Input: part model. Units: mm. Frame: model coordinates. A direction names the side the tool comes from. Round coordinates to 2 decimals unless told otherwise and drop trailing zeros. Write each loop counter-clockwise with the first axis right and the second up, starting at its lowest first coordinate (ties: lowest second). Pieces come first, ordered by that corner, then holes. Notation, with made-up numbers: M 30,71.25 L 89,71.25 A37 cw 89,110.25 Z; hole C 63.25,23.25 d9. An arc over 180 degrees is marked long. Answer as CSV lines item,"result". Start each with the question number.
```python
from build123d import *

# Parameters (mm, degrees)
F1_DEPTH      = 2
F2_R          = 1.663036
F3_DEPTH      = 1
F3_DEPTH_BACK = 2


with BuildPart() as f1:
    # F0 (on Top) → F1 (new body)
    with BuildSketch(Plane.XY):
        with BuildLine():
            ThreePointArc((1.001429, 6.28096), (0.788002, 3.471218), (-1.041486, 1.328047))
            ThreePointArc((-1.041486, 1.328047), (-2.870973, 3.471218), (-3.0844, 6.28096))
            ThreePointArc((-3.0844, 6.28096), (-3.50476, 7.432811), (-4.6266, 6.937897))
            ThreePointArc((-4.6266, 6.937897), (-4.499632, 3.128719), (-2.323149, 0))
            ThreePointArc((-2.323149, 0), (-4.499632, -3.128719), (-4.6266, -6.937897))
            ThreePointArc((-4.6266, -6.937897), (-3.50476, -7.432811), (-3.0844, -6.28096))
            ThreePointArc((-3.0844, -6.28096), (-2.870973, -3.471218), (-1.041486, -1.328047))
            ThreePointArc((-1.041486, -1.328047), (0.788002, -3.471218), (1.001429, -6.28096))
            ThreePointArc((1.001429, -6.28096), (1.421789, -7.432811), (2.543628, -6.937897))
            ThreePointArc((2.543628, -6.937897), (2.416661, -3.128719), (0.240178, 0))
            ThreePointArc((0.240178, 0), (2.416661, 3.128719), (2.543628, 6.937897))
            ThreePointArc((2.543628, 6.937897), (1.421789, 7.432811), (1.001429, 6.28096))
        make_face()
    extrude(amount=F1_DEPTH)

    # F2 (on face) → F3 (join, two sides)
    with BuildSketch(Plane.XY.offset(2)) as f3_sk:
        with Locations((-1.041486, 0)):
            Circle(F2_R)
    extrude(amount=F3_DEPTH)
    extrude(f3_sk.sketch, amount=-F3_DEPTH_BACK)


solid = f1.part
```
Item 1: Cut plane A-A, the plane y = 5. Return loops of the section in (x, z).
Item 2: Cut plane D-D, the plane y = -5.25. Return loops of the section in (x, z).
Item 3: Access query for faces 4 (the face through (-2.97, -3.74, 0.99)), 5 (the face through (-4.583, 3.4, 0.986)). Directions: +Z, -Z, +X, -X, +Y, -Y. A direction counts if a zero-diameter tool reaches every point of the face in a straight line with its end or side. Return the directions, or none.
Item 4: Cut plane C-C, the plane z = 2.25. Return loops of the section in (x, y).
Item 5: Pin query (flat end, axial travel): pin 1 Ø1.7 at (x, y) = (2, 5) entering from +Z; pin 2 Ø2 at (x, y) = (-0.5, 2) entering from +Z. Return the tip coordinate at first contact, or that it passes through.
Item 6: Line query: line 1 (X direction, y = -5, z = 0.15); line 2 (X direction, y = -2.5, z = 1.9); line 3 (Z direction, x = -3.25, y = 6). Output: solid intervals per line, ascending. Write a range as [from, to].
Item 7: Cut plane B-B, the plane x = -1.75. Return loops of the section in (y, z), plus the area to 3 significant figures.
Item 8: Draft query along Y for faces 1 (the face through (-4.555, -3.302, 0.986)), 2 (the face through (0.89, 3.74, 0.99)), 3 (the face through (-4, -4, 2)). Return one class per face: +Y half, -Y half, draft (parallel to the pull), parting line (faces both ways), or undercut.
Results list:
1,outline,"M -4.84,0 L -3.21,0 L -3.21,2 L -4.84,2 Z; M 1.13,0 L 2.75,0 L 2.75,2 L 1.13,2 Z"
2,outline,"M -4.84,0 L -3.21,0 L -3.21,2 L -4.84,2 Z; M 1.13,0 L 2.76,0 L 2.76,2 L 1.13,2 Z"
3,face 4,"+Z, -Z"
3,face 5,"+Z, -Z, -X"
4,outline,"C -1.04,0 d3.33"
5,pin 1,"z = 2"
5,pin 2,"z = 3"
6,line 1,"[-4.84, -3.21], [1.13, 2.75]"
6,line 2,"[-4.26, -2.32], [0.24, 2.17]"
6,line 3,"[0, 2]"
7,outline,"M -1.86,0 L 1.86,0 L 1.86,2 L 1.5,2 L 1.5,3 L -1.5,3 L -1.5,2 L -1.86,2 Z"
7,area,"10.5 mm²"
8,face 1,"undercut"
8,face 2,"undercut"
8,face 3,"draft"
